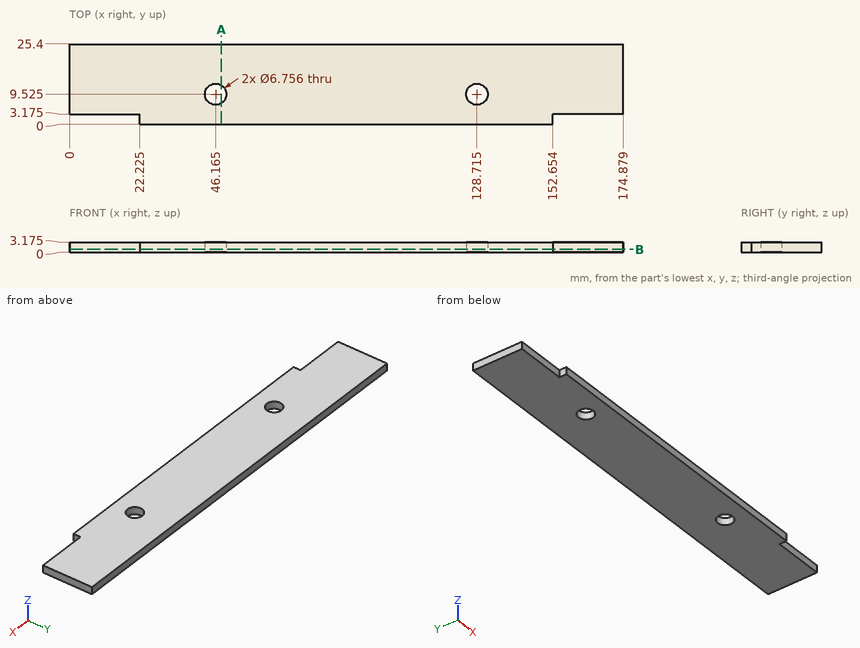
Print and shaded views of the part. All mm, measured from the part's lowest x, y and z. Coordinates: 2 decimals unless noted, no trailing zeros. Loops run counter-clockwise (first coordinate to the right, second up) from the corner with the lowest first, then second, coordinate; pieces in that order, holes last. Notation, with made-up numbers: (15, 82) -> (20, 82) arc R10 ccw to (20, 100) -> close; hole circle Ø5 at (68.25, 30). An arc over 180 degrees is marked (long way). Use one line per item in the form item = value. Start each with the question number.
(1) Cut at B-B on z = 0.95. Give the cut face in (x, y) (1 decimal).
(2) Flat gauge pins, fed straight in: pin 1 (8 mm diameter, centred on x = 128.71, y = 9.52, fed in from -Z); pin 2 (1.6 mm diameter, centred on y = 1, z = 2, fed in from -X) (1 decimal). Where does each tip first touch, or does it go through?
(3) Probe probe 1 along X at (y, z) = (10, 2.85); probe 2 along X at (y, z) = (6.5, 0.6) (1 decimal); probe 3 along Y at (x, z) = (21, 1.9) (1 decimal). List the from-to ranges inside material, lowest first. Write a range as from..to.
(4) Cut at A-A on x = 48. Give the cut face in (y, z) (1 decimal).
Values:
q1.outline = (0, 3.2) -> (22.2, 3.2) -> (22.2, 0) -> (152.7, 0) -> (152.7, 3.2) -> (174.9, 3.2) -> (174.9, 25.4) -> (0, 25.4) -> close; hole circle Ø6.8 at (46.2, 9.5); hole circle Ø6.8 at (128.7, 9.5)
q2.pin_1 = 0
q2.pin_2 = 22.2
q3.probe_1 = 0..42.82, 49.51..125.37, 132.06..174.88
q3.probe_2 = 0..44.7, 47.7..127.2, 130.2..174.9
q3.probe_3 = 3.2..25.4
q4.outline = (0, 0) -> (6.7, 0) -> (6.7, 3.2) -> (0, 3.2) -> close; (12.4, 0) -> (25.4, 0) -> (25.4, 3.2) -> (12.4, 3.2) -> close
